from build123d import *

# Parameters (mm, degrees)
SKETCH_1_W                  = 200
SKETCH_1_H                  = 200
EXTRUDE_1_DEPTH             = 12
SKETCH_2_R                  = 11
CUT_EXTRUDE_2_DEPTH         = 284.097156468
PATTERN_LINEAR_1_COUNT      = 2
PATTERN_LINEAR_1_PITCH      = 125
PATTERN_LINEAR_1_COUNT_DIR2 = 2
PATTERN_LINEAR_1_PITCH_DIR2 = 125
SKETCH_3_W                  = 320
SKETCH_3_H                  = 20
EXTRUDE_3_DEPTH             = 100
CUT_EXTRUDE_4_DEPTH         = 304.716973513
SKETCH_6_R                  = 11
CUT_EXTRUDE_6_DEPTH         = 304.716973513
PATTERN_LINEAR_3_COUNT      = 3
PATTERN_LINEAR_3_PITCH      = 122


with BuildPart() as part:
    # 草图1 → 拉伸1 (new body)
    with BuildSketch(Plane.XY):
        with Locations((100, 100)):
            Rectangle(SKETCH_1_W, SKETCH_1_H)
    extrude(amount=EXTRUDE_1_DEPTH)

    # 草图2 → 拉伸2 (cut, through all)
    with BuildSketch(Plane.XY.offset(12)):
        with Locations((37.5, 37.5)):
            Circle(SKETCH_2_R)
    cut_extrude_2 = extrude(amount=-CUT_EXTRUDE_2_DEPTH, mode=Mode.SUBTRACT)

    # 阵列(线性)1: Cut-Extrude 2 2 × 2
    with Locations(*[(i * PATTERN_LINEAR_1_PITCH, j * PATTERN_LINEAR_1_PITCH_DIR2, 0) for i in range(PATTERN_LINEAR_1_COUNT) for j in range(PATTERN_LINEAR_1_COUNT_DIR2) if (i, j) != (0, 0)]):
        add(cut_extrude_2, mode=Mode.SUBTRACT)

    # 草图3 → 拉伸3 (add)
    with BuildSketch(Plane.XY.offset(12)):
        with Locations((100, 100)):
            Rectangle(SKETCH_3_W, SKETCH_3_H)
    extrude(amount=EXTRUDE_3_DEPTH)

    # 草图4 → 拉伸4 (cut, through all)
    with BuildSketch(Plane.XZ.offset(-90)):
        Polygon((200, 12), (260, 42), (260, 12), align=None)
        Polygon((-60, 42), (0, 12), (-60, 12), align=None)
    extrude(amount=-CUT_EXTRUDE_4_DEPTH, mode=Mode.SUBTRACT)

    # 草图6 → 拉伸6 (cut, through all)
    with BuildSketch(Plane.XZ.offset(-90)):
        with Locations(Location((-22, 68, 0), (0, 0, 270))):
            Circle(SKETCH_6_R)
    cut_extrude_6 = extrude(amount=-CUT_EXTRUDE_6_DEPTH, mode=Mode.SUBTRACT)

    # 阵列(线性)3: 拉伸6 ×3
    with Locations(*[(i * PATTERN_LINEAR_3_PITCH, 0, 0) for i in range(1, PATTERN_LINEAR_3_COUNT)]):
        add(cut_extrude_6, mode=Mode.SUBTRACT)


solid = part.part
Source: CAD feature listing. Evaluate the final solid. Frame: model axes, mm. A direction names the side the tool comes from. Give positions to 0.01 mm unless a question says otherwise; leave off trailing zeros. Write each loop counter-clockwise with the first axis right and the second up, starting at its lowest first coordinate (ties: lowest second). Pieces come first, ordered by that corner, then holes. Notation, with made-up numbers: M 81.25,-9.75 L 139.25,-9.75 A4 cw 139.25,-3.75 Z; hole C 84,13 d3. An arc over 180 degrees is marked long. Return JSON: item names as keys, results as strings. Group by question number.
1) Cut plane D-D, the plane x = 162.5. Output: boundary loops of the cut face in (y, z).
2) Cut plane A-A, the plane x = 222. Output: boundary loops of the cut face in (y, z).
3) Pull-direction query (Z, two-part tool) for faces 4 (the face through (-22, 100, 79)), 5 (the face through (99, 46, 12)), 6 (the face through (99, 200, 6)); classes: pulls with the +Z half, pulls with the -Z half, needs draft (parallel to the pull), parting line crosses it, or undercut.
4) Cut plane B-B, the plane y = 37.5. Output: boundary loops of the cut face in (x, z).
5) Material intervals for line 1 along Y through (x, z) = (162.5, 4); line 2 along X through (y, z) = (103.25, 68); line 3 along Z through (x, y) = (45.5, 121), sorted ascending. Write a range as [from, to].
6) Cut plane C-C, the plane z = 68. Output: boundary loops of the cut face in (x, y).
7) Set-up query: faces 1 (the face through (230, 100, 27)), 2 (the face through (98, 110, 50)), 3 (the face through (98, 90, 50)). Return all of +Z, -Z, +X, -X, +Y, -Y with unobstructed straight access to the full face (end or side cutting, diameter ignored); none if empty.
8) Pin query (flat end, axial travel): P1, Ø10, axis at x = -8.5, z = 100, coming from the -Y side; P2, Ø1, axis at x = 36, z = 33.5, coming from the +Y side; P3, Ø17.5, axis at x = -22, z = 68, coming from the -Y side; P4, Ø9.5, axis at y = 130.5, z = 6.5, coming from the -X side. Return the tip coordinate at first contact, or that it passes through.
Recorded:
{
 "1": {"outline": "M 0,0 L 26.5,0 L 26.5,12 L 0,12 Z; M 48.5,0 L 151.5,0 L 151.5,12 L 110,12 L 110,112 L 90,112 L 90,12 L 48.5,12 Z; M 173.5,0 L 200,0 L 200,12 L 173.5,12 Z"},
 "2": {"outline": "M 90,23 L 110,23 L 110,57 L 90,57 Z; M 90,79 L 110,79 L 110,112 L 90,112 Z"},
 "3": {"face 4": "undercut", "face 5": "pulls with the +Z half", "face 6": "needs draft"},
 "4": {"outline": "M 0,0 L 26.5,0 L 26.5,12 L 0,12 Z; M 48.5,0 L 151.5,0 L 151.5,12 L 48.5,12 Z; M 173.5,0 L 200,0 L 200,12 L 173.5,12 Z"},
 "5": {"line 1": "y = [0, 26.5], [48.5, 151.5], [173.5, 200]", "line 2": "x = [-60, -33], [-11, 89], [111, 211], [233, 260]", "line 3": "z = [0, 12]"},
 "6": {"outline": "M -60,90 L -33,90 L -33,110 L -60,110 Z; M -11,90 L 89,90 L 89,110 L -11,110 Z; M 111,90 L 211,90 L 211,110 L 111,110 Z; M 233,90 L 260,90 L 260,110 L 233,110 Z"},
 "7": {"face 1": "-Z, +X, +Y, -Y", "face 2": "+Z, +X, -X, +Y", "face 3": "+Z, +X, -X, -Y"},
 "8": {"P1": "stops at y = 90", "P2": "stops at y = 110", "P3": "passes through", "P4": "stops at x = 0"}
}
